Read the model definition and answer for the solid it produces. Units are mm, in the model's axes. A direction names the side the tool comes from. Give positions to 0.01 mm unless a question says otherwise; leave off trailing zeros. Loops run counter-clockwise (first coordinate to the right, second up) from the corner with the lowest first, then second, coordinate; pieces in that order, holes last. Notation, with made-up numbers: (-28.75, 21) - (-18.75, 21) arc R28 cw to (-18.75, 53) - close; hole circle Ø8 at (-27.5, -36). An arc over 180 degrees is marked (long way). Write item = value, one per line. Start each with the question number.
from build123d import *

# Parameters (mm, degrees)
F0_W     = 240
F0_H     = 20
F2_W     = 40
F2_H     = 120
F3_DEPTH = 40
F4_R     = 19.99999
F5_W     = 100
F5_H     = 20


# Not quite as in the source:
# - a fillet or chamfer is up to 0.001 mm smaller than in the source, because OpenCascade refuses the exact size


with BuildPart() as f1:
    # F0 (on Right) → F1 (revolve)
    with BuildSketch(Plane.YZ):
        with Locations((0, 10)):
            Rectangle(F0_W, F0_H)
    revolve(axis=Axis((0, 0, 0), (0, 1, 0)))

    # F2 (on Top) → F3 (join)
    with BuildSketch(Plane.XY):
        Rectangle(F2_W, F2_H)
    extrude(amount=-F3_DEPTH)

    # F4 (radius 20 in the source; OpenCascade refuses exactly that, so slightly less here)
    f4_edges = [f1.edges().sort_by_distance(p)[0] for p in [
        (0, -60, -40),
        (0, 60, -40),
    ]]
    fillet(f4_edges, radius=F4_R)

    # F5 (on Front) → F6 (revolve)
    with BuildSketch(Plane.XZ):
        with Locations((0.1484978533, -50)):
            Rectangle(F5_W, F5_H)
    revolve(axis=Axis((43.9392195031, 0, -40), (1, 0, 0)))


solid = f1.part
1. Consider line 1 along X through (y, z) = (-29.5, -18); line 2 along Z through (x, y) = (31.5, 4.5); line 3 along Y through (x, z) = (22.5, -40.5). Determine where each line is inside the solid, lowest interval first. Write a range as [from, to].
2. Given P1, Ø10, axis at x = 0.5, y = 22, coming from the -Z side; P2, Ø10, axis at y = -69, z = -12, coming from the +X side (3 decimals); P3, Ø1, axis at x = 6, z = -49.5, coming from the -Y side, each flat-ended and moving along its own axis, determine where each tip first touches the part or whether it passes through.
3. A cutting plane is placed at C-C on z = -10.5. Give the vertices of the cut face in (x, y), and give its area (3 significant figures).
4. A cutting plane is placed at D-D on y = 102. Give the vertices of the cut face in (x, z).
5. A tool of negligible diameter and unlimited length cuts with its end or side. For faces 1 (the flat face through (5.8, 60, -19.6)), 2 (the flat face through (20, -1, -15)), 3 (the cylindrical face through (-7.66, 1.68, 18.475)), 4 (the flat face through (0, 30, -40)), 5 (the flat face through (5.8, -60, -19.6)), from which of +Z, -Z, +X, -X, +Y, -Y can it reach the whole face along a straight path? Write none if from no direction.
6. A cutting plane is placed at B-B on y = 0. Give the vertices of the cut face in (x, z).
Reply:
q1.line_1 = [-20, 20]
q1.line_2 = [-59.49, -20.51]
q1.line_3 = [-19.99, 19.99]
q2.P1 = -50.54
q2.P2 = 18.735
q2.P3 = -17.86
q3.outline = (-20, -60) - (-17.02, -60) - (-17.02, -120) - (17.02, -120) - (17.02, -60) - (20, -60) - (20, 60) - (17.02, 60) - (17.02, 120) - (-17.02, 120) - (-17.02, 60) - (-20, 60) - close
q3.area = 8,890 mm^2
q4.outline = circle Ø40 at (0, 0)
q5.face_1 = -Z, +Y
q5.face_2 = +Z, +X
q5.face_3 = none
q5.face_4 = -Z, +X, -X, +Y
q5.face_5 = -Z, -Y
q6.outline = (-49.85, -60) - (50.15, -60) - (50.15, -20) - (20, -20) - (20, 0) arc R20 ccw to (-20, 0) - (-20, -20) - (-49.85, -20) - close
